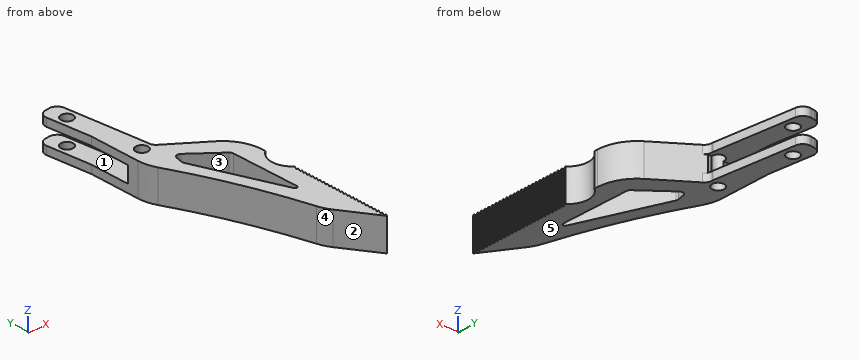
```python
from build123d import *

# Parameters (mm, degrees)
BOSS_EXTRUDE1_DEPTH     = 4
SKETCH2_W               = 20
SKETCH2_H               = 25
CUT_EXTRUDE1_DEPTH      = 2
CUT_EXTRUDE2_DEPTH      = 1
CUT_EXTRUDE2_DEPTH_BACK = 9
CUT_EXTRUDE3_DEPTH      = 9
LPATTERN2_COUNT         = 26
LPATTERN2_PITCH         = 1.0025
CUT_EXTRUDE4_DEPTH      = 9
CUT_EXTRUDE5_DEPTH      = 9
FILLET1_R               = 10
FILLET2_R               = 2
FILLET3_R               = 1
FILLET4_R               = 0.5
SKETCH7_R               = 1.5
CUT_EXTRUDE6_DEPTH      = 9.0000001


with BuildPart() as part:
    # Sketch1 → Boss-Extrude1 (new body, symmetric)
    with BuildSketch(Plane.XY):
        Polygon((0, 0), (-20, 30.005392849), (-20, 60.135392849), (-21.435566599, 73.055886204), (-16.466146078, 73.608027203), (-14.000284373, 51.414595156), (-14.000284373, 50.014595156), (0, 40.028289364), align=None)
    extrude(amount=BOSS_EXTRUDE1_DEPTH, both=True)

    # Sketch2 → Cut-Extrude1 (cut, symmetric)
    with BuildSketch(Plane.XY):
        with Locations((-24.000284373, 62.514595156)):
            Rectangle(SKETCH2_W, SKETCH2_H)
    extrude(amount=CUT_EXTRUDE1_DEPTH, both=True, mode=Mode.SUBTRACT)

    # Sketch3 → Cut-Extrude2 (cut, two sides)
    with BuildSketch(Plane.XY.offset(4)) as cut_extrude2_sk:
        with BuildLine():
            Line((91.496624596, 102.650757811), (0, 34.028289364))
            ThreePointArc((0, 34.028289364), (-2, 30.028289364), (0, 26.028289364))
            Line((0, 26.028289364), (91.496624596, -42.594179083))
            Line((91.496624596, -42.594179083), (320.238186086, -42.594179083))
            Line((320.238186086, -42.594179083), (320.238186086, 102.650757811))
            Line((320.238186086, 102.650757811), (91.496624596, 102.650757811))
        make_face()
    extrude(amount=CUT_EXTRUDE2_DEPTH, mode=Mode.SUBTRACT)
    extrude(cut_extrude2_sk.sketch, amount=-CUT_EXTRUDE2_DEPTH_BACK, mode=Mode.SUBTRACT)

    # Sketch4 → Cut-Extrude3 (cut, through all)
    with BuildSketch(Plane.XY.offset(4)):
        Polygon((0, 26.028289364), (-0.5, 25.028289364), (0, 25.028289364), align=None)
    cut_extrude3 = extrude(amount=-CUT_EXTRUDE3_DEPTH, mode=Mode.SUBTRACT)

    # LPattern2: Cut-Extrude3 ×26
    with Locations(*[(0, -i * LPATTERN2_PITCH, 0) for i in range(1, LPATTERN2_COUNT)]):
        add(cut_extrude3, mode=Mode.SUBTRACT)

    # Sketch5 → Cut-Extrude4 (cut, through all)
    with BuildSketch(Plane.XY.offset(4)):
        with BuildLine():
            Line((-20, 30.005392849), (-6.955074875, 10.434487696))
            ThreePointArc((-6.955074875, 10.434487696), (-12.476218242, 28.097776313), (-20, 45.005392849))
            Line((-20, 45.005392849), (-20, 30.005392849))
        make_face()
    extrude(amount=-CUT_EXTRUDE4_DEPTH, mode=Mode.SUBTRACT)

    # Sketch6 → Cut-Extrude5 (cut, through all)
    with BuildSketch(Plane.XY.offset(4)):
        with BuildLine():
            Line((-13.544369657, 44.932398873), (-5.010201765, 37.897373757))
            Line((-5.010201765, 37.897373757), (-4.779170601, 17.572398873))
            add(Edge.make_bspline(
                [(-4.779170601, 17.572398873), (-14.345858132, 41.272398873)],
                knots=[0, 0, 1, 1], degree=1))
            Line((-14.345858132, 41.272398873), (-13.544369657, 44.932398873))
        make_face()
    extrude(amount=-CUT_EXTRUDE5_DEPTH, mode=Mode.SUBTRACT)

    # Fillet1
    fillet1_edges = [part.edges().sort_by_distance(p)[0] for p in [
        (0, 40.028289364, 0),
        (-20, 45.005392849, 0),
        (-6.955074875, 10.434487696, 0),
    ]]
    fillet(fillet1_edges, radius=FILLET1_R)

    # Fillet2
    fillet2_edges = [part.edges().sort_by_distance(p)[0] for p in [
        (-21.435566599, 73.055886204, 3),
        (-16.466146078, 73.608027203, 3),
        (-14.000284373, 50.014595156, 3),
        (-21.435566599, 73.055886204, -3),
        (-16.466146078, 73.608027203, -3),
        (-14.000284373, 50.014595156, -3),
    ]]
    fillet(fillet2_edges, radius=FILLET2_R)

    # Fillet3
    fillet3_edges = [part.edges().sort_by_distance(p)[0] for p in [
        (-14.345858132, 41.272398873, 0),
        (-5.010201765, 37.897373757, 0),
        (-13.544369657, 44.932398873, 0),
    ]]
    fillet(fillet3_edges, radius=FILLET3_R)

    # Fillet4
    fillet4_edges = [part.edges().sort_by_distance(p)[0] for p in [
        (-4.779170601, 17.572398873, 0),
    ]]
    fillet(fillet4_edges, radius=FILLET4_R)

    # Sketch7 → Cut-Extrude6 (cut, through all)
    with BuildSketch(Plane.XY.offset(4)):
        with Locations((-18.416383851, 68.521557639)):
            Circle(SKETCH7_R)
        with Locations((-16.381192126, 50.204273598)):
            Circle(SKETCH7_R)
    extrude(amount=-CUT_EXTRUDE6_DEPTH, mode=Mode.SUBTRACT)


solid = part.part
```
Read the model definition and answer for the solid it produces. Units are mm, in the model's axes. Face numbers are marked on the shaded views. A direction names the side the tool comes from. Round coordinates to 2 decimals unless told otherwise and drop trailing zeros. Loops run counter-clockwise (first coordinate to the right, second up) from the corner with the lowest first, then second, coordinate; pieces in that order, holes last. Notation, with made-up numbers: (82.25, 37.25) -> (91.25, 37.25) arc R5 ccw to (91.25, 43.25) -> close; hole circle Ø6 at (61.5, -26.5). An arc over 180 degrees is marked (long way). One line per item, written item: value.
1) Flat-ended cylindrical pins translate along their axes: P1, Ø0.6, axis at x = -0.5, z = -1, coming from the +Y side; P2, Ø1.5, axis at y = 50, z = 0, coming from the +X side. Find the tip coordinate at first contact, or state that the pin passes through.
Answer list:
P1: stops at y = 38.8
P2: stops at x = -12.93
2) A cutting plane is placed at C-C (z = 3). Give the number of separate pieces and of enclosed holes in the cut face, and give its area (3 significant figures).
Answer list:
separate pieces: 1
enclosed holes: 3
area: 480 mm²
3) Consider L1, parallel to X at y = 42, z = -1.5; L2, parallel to X at y = 29.5, z = 3.25; L3, parallel to Y at x = -5.25, z = -1. Determine where each line is inside the solid, lowest interval first. Write a range as [from, to].
Answer list:
L1: x = [-18.49, -14.19], [-9.99, -2.98]
L2: x = [-13.01, -9.59], [-4.91, -1.97]
L3: y = [7.88, 19.73], [38.08, 43.77]
4) For the marked faces 1 and 2, determine the directions among +Z, -Z, +X, -X, +Y, -Y from which every point of the face is accessible in a straight line to the end or side of a thin tool.
Answer list:
face 1: +X, -X, +Y
face 2: +Z, -Z, -X, -Y
5) A cutting plane is placed at B-B (y = 52.5). Determine the outline of the cut face in (x, z), and give its area (3 significant figures).
Answer list:
outline: (-20, -4) -> (-14.12, -4) -> (-14.12, -2) -> (-20, -2) -> close; (-20, 2) -> (-14.12, 2) -> (-14.12, 4) -> (-20, 4) -> close
area: 23.5 mm²
6) A cutting plane is placed at A-A (y = 64.5). Determine the outline of the cut face in (x, z), and give its area (3 significant figures).
Answer list:
outline: (-20.48, -4) -> (-15.45, -4) -> (-15.45, -2) -> (-20.48, -2) -> close; (-20.48, 2) -> (-15.45, 2) -> (-15.45, 4) -> (-20.48, 4) -> close
area: 20.1 mm²
7) The mould has two halves that part along X. Classify the marked faces 3, 4 and 5: pulls with the +X half, pulls with the -X half, needs draft (parallel to the pull), parting line crosses it, or undercut.
Answer list:
face 3: undercut
face 4: pulls with the -X half
face 5: needs draft
